Autodesk Inventor part; units mm, degrees
ref_plane "YZ Plane" through (0, 0, 0) normal (1, 0, 0) x (0, 1, 0)
ref_plane "XZ Plane" through (0, 0, 0) normal (0, 1, 0) x (-1, 0, 0)
ref_plane "XY Plane" through (0, 0, 0) normal (0, 0, 1) x (1, 0, 0)
sketch "Sketch1" plane through (0, 0, 0) normal (0, 0, 1) x (1, 0, 0)
  line L0 (1.016, 0) -> (4.064, 0)
  line L1 (5.08, -1.016) -> (5.08, -1.016)
  line L2 (4.064, -2.032) -> (1.016, -2.032)
  line L3 (0, -1.016) -> (0, -1.016)
  line L4 (1.016, -3.81) -> (4.064, -3.81)
  line L5 (6.858, -1.016) -> (6.858, -1.016)
  line L6 (4.064, 1.778) -> (1.016, 1.778)
  line L7 (-1.778, -1.016) -> (-1.778, -1.016)
  arc A0 (6.858, -1.016) -> (4.064, 1.778) centre (4.064, -1.016) ccw
  arc A1 (4.064, -3.81) -> (6.858, -1.016) centre (4.064, -1.016) ccw
  arc A2 (5.08, -1.016) -> (4.064, 0) centre (4.064, -1.016) ccw
  arc A3 (4.064, -2.032) -> (5.08, -1.016) centre (4.064, -1.016) ccw
  arc A4 (1.016, 0) -> (0, -1.016) centre (1.016, -1.016) ccw
  arc A5 (0, -1.016) -> (1.016, -2.032) centre (1.016, -1.016) ccw
  circle A6 centre (-9.144, -1.016) radius 2.286
  circle A7 centre (-9.144, -1.016) radius 0.762
  arc A8 (1.016, 1.778) -> (-1.778, -1.016) centre (1.016, -1.016) ccw
  arc A9 (-1.778, -1.016) -> (1.016, -3.81) centre (1.016, -1.016) ccw
  arc A10 (-8.8323, 1.2486) -> (0.3651, 1.7011) centre (-5.4362, 25.9197) ccw
  arc A11 (0.3651, -3.7331) -> (-8.8323, -3.2806) centre (-5.4362, -27.9517) ccw
  line L8 (-8.0967, 1.016) -> (-0.9017, 1.016) construction
  line L9 (-8.0967, -3.048) -> (-0.9017, -3.048) construction
  line L10 (-6.858, -1.016) -> (-1.778, -1.016) construction
  point P0 (0, 0)
  point P1 (5.08, -2.032)
  point P2 (5.08, 0)
  point P3 (0, -2.032)
  point P4 (6.858, -3.81)
  point P5 (6.858, 1.778)
  point P6 (-8.382, -1.016)
  point P7 (5.08, -1.016)
  dimension "d15" = 1.524
  dimension "d0" = 5.08
  dimension "d1" = 2.032
  dimension "d2" = 1.778
  dimension "d3" = 5.588
  dimension "d4" = 2.794
  dimension "d5" = 2.794
  dimension "d6" = 1.016
  dimension "d8" = 1.524
  dimension "d9" = 2.794
  dimension "d10" = 8.382
  dimension "d11" = 4.064
  dimension "d12" = 2.032
extrude "Extrusion1" add sketch "Sketch1" along normal blind 1.778
properties part number "Elbow holder" material "Phenolic Resin"
Input: part model. Units: mm. Frame: model coordinates. A direction names the side the tool comes from. Give positions to 0.01 mm unless a question says otherwise; leave off trailing zeros. Order: outer loops, then holes, each group sorted by start corner. A loop starts at its lowest first (then second) coordinate and runs counter-clockwise, first axis right, second up. Notation, with made-up numbers: (-35, 42.25) -> (-8, 42.25) arc R32 ccw to (-8, 81.25) -> close; hole circle Ø3 at (78, 30.5). An arc over 180 degrees is marked (long way). Use one line per item in the form item = value.
1) Reachability of faces 1 (the flat face through (3, -3.81, 1)), 2 (the cylindrical face through (0, -1, 1)) from +Z, -Z, +X, -X, +Y, -Y: full face, straight path, thin tool, end or side. Return the list, or none.
Response values:
face_1 = +Z, -Z, +X, -X, -Y
face_2 = +Z, -Z
2) Section C-C, the plane z = 0.55. Return loops of the section in (x, y), and give its area (3 significant figures).
Response values:
outline = (-8.83, -3.28) arc R24.9 cw to (0.37, -3.73) arc R2.79 ccw to (1.02, -3.81) -> (4.06, -3.81) arc R2.79 ccw to (4.06, 1.78) -> (1.02, 1.78) arc R2.79 ccw to (0.37, 1.7) arc R24.9 cw to (-8.83, 1.25) arc R2.29 ccw (long way) to start; hole circle Ø1.52 at (-9.14, -1.02); hole (1.02, -2.03) -> (4.06, -2.03) arc R1.02 ccw to (4.06, 0) -> (1.02, 0) arc R1.02 ccw to start
area = 71.8 mm^2
3) Section B-B, the plane y = -0.7. Return loops of the section in (x, z).
Response values:
outline = (-11.41, 0) -> (-9.84, 0) -> (-9.84, 1.78) -> (-11.41, 1.78) -> close; (-8.45, 0) -> (0.05, 0) -> (0.05, 1.78) -> (-8.45, 1.78) -> close; (5.03, 0) -> (6.84, 0) -> (6.84, 1.78) -> (5.03, 1.78) -> close
4) Section D-D, the plane x = -9.25. Return loops of the section in (y, z), and give its area (3 significant figures).
Response values:
outline = (-3.3, 0) -> (-1.77, 0) -> (-1.77, 1.78) -> (-3.3, 1.78) -> close; (-0.26, 0) -> (1.27, 0) -> (1.27, 1.78) -> (-0.26, 1.78) -> close
area = 5.44 mm^2
5) First-contact query: pin 1 Ø2.5 at (x, y) = (-9.144, -1.016) entering from +Z. Flat tip, straight axial feed; report the tip coordinate or a pass-through.
Response values:
pin_1 = 1.78
6) Section A-A, the plane x = 1.25. Return loops of the section in (y, z).
Response values:
outline = (-3.81, 0) -> (-2.03, 0) -> (-2.03, 1.78) -> (-3.81, 1.78) -> close; (0, 0) -> (1.78, 0) -> (1.78, 1.78) -> (0, 1.78) -> close
7) Line query: probe 1 along X at (y, z) = (-0.95, 0.4); probe 2 along Y at (x, z) = (2.5, 0.25); probe 3 along X at (y, z) = (-1.5, 1.4). Output: solid intervals per line, ascending.
Response values:
probe_1 = -11.43 to -9.9, -8.38 to 0, 5.08 to 6.86
probe_2 = -3.81 to -2.03, 0 to 1.78
probe_3 = -11.38 to -9.73, -8.56 to 0.12, 4.96 to 6.82
8) Mould query, pull axis X, two halves, no side actions, for faces 3 (the cylindrical face through (-4.277, -3.075, 0.877)), 4 (the flat face through (-2, -1, 0)), 5 (the cylindrical face through (6.857, -0.955, 0.877)). Classes: pulls with the +X half, pulls with the -X half, needs draft (parallel to the pull), parting line crosses it, or undercut.
Response values:
face_3 = undercut
face_4 = needs draft
face_5 = pulls with the +X half
